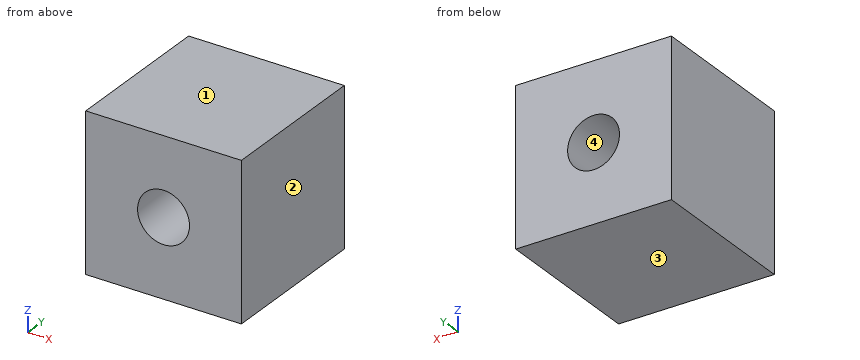
```python
from build123d import *

# Parameters (mm, degrees)
F0_W     = 60
F0_H     = 60
F1_DEPTH = 60
F2_R     = 10
F3_DEPTH = 60.001


with BuildPart() as f1:
    # F0 (on Front) → F1 (new body)
    with BuildSketch(Plane.XZ):
        Rectangle(F0_W, F0_H)
    extrude(amount=F1_DEPTH)

    # F2 (on face) → F3 (cut, through all)
    with BuildSketch(Plane.XZ.offset(60)):
        Circle(F2_R)
    extrude(amount=-F3_DEPTH, mode=Mode.SUBTRACT)


solid = f1.part
```
Verification items for the finished model (mm, model axes). Face numbers are marked on the shaded views. Give positions to 0.01 mm unless a question says otherwise; leave off trailing zeros. Order: outer loops, then holes, each group sorted by start corner. A loop starts at its lowest first (then second) coordinate and runs counter-clockwise, first axis right, second up. Notation, with made-up numbers: M 35,4.25 L 49,4.25 A23 ccw 49,13.25 Z; hole C 57,2.5 d3. An arc over 180 degrees is marked long. Answer in a Markdown table with one row per item. Add a question column.
Item 1: Mould release check, pull along Z, two halves, no side actions. Record for the marked faces 1, 2, 3 and 4: released by +Z, released by -Z, zero draft, split by the parting line, or undercut.
Item 2: Section check C-C, the plane y = -53. Enter the section's corners in (x, z), and give its area (3 significant figures).
Item 3: Scan lines: probe 1 along Z at (x, y) = (0, -41); probe 2 along X at (y, z) = (-10, -1.5); probe 3 along X at (y, z) = (-30.5, 7). Record each from-to range of solid material in increasing order. Write a range as from..to.
Item 4: Section check A-A, the plane z = 0. Enter the section's corners in (x, y), and give its area (3 significant figures).
Item 5: Section check B-B, the plane x = 0. Enter the section's corners in (y, z), and give its area (3 significant figures).
Filled sheet:
| question | item | result |
|---|---|---|
| 1 | face 1 | released by +Z |
| 1 | face 2 | zero draft |
| 1 | face 3 | released by -Z |
| 1 | face 4 | undercut |
| 2 | outline | M -30,-30 L 30,-30 L 30,30 L -30,30 Z; hole C 0,0 d20 |
| 2 | area | 3,290 mm^2 |
| 3 | probe 1 | z = -30..-10, 10..30 |
| 3 | probe 2 | x = -30..-9.89, 9.89..30 |
| 3 | probe 3 | x = -30..-7.14, 7.14..30 |
| 4 | outline | M -30,-60 L -10,-60 L -10,0 L -30,0 Z; M 10,-60 L 30,-60 L 30,0 L 10,0 Z |
| 4 | area | 2,400 mm^2 |
| 5 | outline | M -60,-30 L 0,-30 L 0,-10 L -60,-10 Z; M -60,10 L 0,10 L 0,30 L -60,30 Z |
| 5 | area | 2,400 mm^2 |
